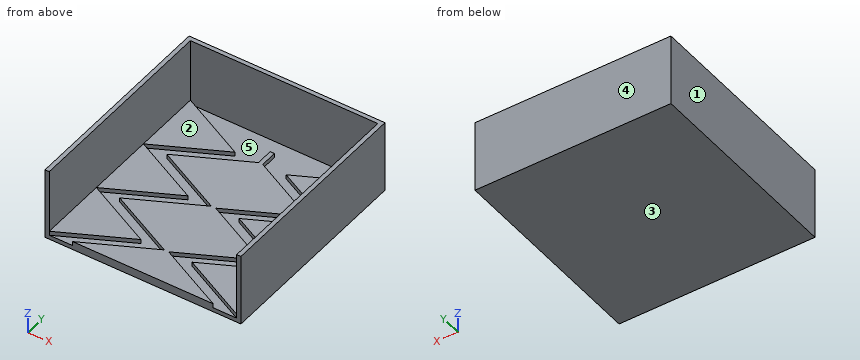
from build123d import *

# Parameters (mm, degrees)
F1_DEPTH = 3.175
F2_DEPTH = 50.8
F3_DEPTH = 3.175


# Not quite as in the source:
# - a length typed as a fraction of an inch, garbled in the dataset ("3 / 203.2 mm" for 3/8 in), is restored


with BuildPart() as f1:
    # F0 (on Top) → F1 (new body)
    with BuildSketch(Plane.XY):
        Polygon((53.975, 25.4), (3.175, 0), (20.638, 0), (71.438, 25.39975), (20.638, 50.7995), (71.438, 76.1995), (20.638, 101.5995), (71.438, 126.9995), (71.438, 139.6995), (74.613, 139.6995), (74.613, 126.9995), (125.412, 101.6), (74.612, 76.2), (125.412, 50.8), (74.612, 25.4), (125.412, 0), (142.875, 0), (92.075, 25.4), (142.875, 50.8), (92.075, 76.2), (142.875, 101.6), (92.075, 127), (142.875, 152.4), (3.175, 152.4), (53.975, 127), (3.175, 101.6), (53.975, 76.2), (3.175, 50.8), align=None)
        Polygon((142.875, 101.6), (142.875, 152.4), (92.075, 127), align=None)
        Polygon((0, 155.575), (0, 0), (3.175, 0), (3.175, 50.8), (3.175, 101.6), (3.175, 152.4), (142.875, 152.4), (142.875, 101.6), (142.875, 50.8), (142.875, 0), (146.05, 0), (146.05, 155.575), align=None)
        Polygon((92.075, 76.2), (142.875, 50.8), (142.875, 101.6), align=None)
        Polygon((92.075, 25.4), (142.875, 0), (142.875, 50.8), align=None)
        Polygon((71.438, 25.39975), (20.638, 0), (125.412, 0), (74.612, 25.4), (125.412, 50.8), (74.612, 76.2), (125.412, 101.6), (74.613, 126.9995), (74.613, 139.6995), (71.438, 139.6995), (71.438, 126.9995), (20.638, 101.5995), (71.438, 76.1995), (20.638, 50.7995), align=None)
        Polygon((3.175, 50.8), (3.175, 0), (53.975, 25.4), align=None)
        Polygon((3.175, 101.6), (3.175, 50.8), (53.975, 76.2), align=None)
        Polygon((3.175, 152.4), (3.175, 101.6), (53.975, 127), align=None)
    extrude(amount=-F1_DEPTH)

    # F0 (on Top) → F2 (join)
    with BuildSketch(Plane.XY):
        Polygon((0, 155.575), (0, 0), (3.175, 0), (3.175, 50.8), (3.175, 101.6), (3.175, 152.4), (142.875, 152.4), (142.875, 101.6), (142.875, 50.8), (142.875, 0), (146.05, 0), (146.05, 155.575), align=None)
    extrude(amount=F2_DEPTH)

    # F0 (on Top) → F3 (join)
    with BuildSketch(Plane.XY):
        Polygon((3.175, 152.4), (3.175, 101.6), (53.975, 127), align=None)
        Polygon((3.175, 101.6), (3.175, 50.8), (53.975, 76.2), align=None)
        Polygon((3.175, 50.8), (3.175, 0), (53.975, 25.4), align=None)
        Polygon((92.075, 25.4), (142.875, 0), (142.875, 50.8), align=None)
        Polygon((92.075, 76.2), (142.875, 50.8), (142.875, 101.6), align=None)
        Polygon((142.875, 101.6), (142.875, 152.4), (92.075, 127), align=None)
        Polygon((71.438, 25.39975), (20.638, 0), (125.412, 0), (74.612, 25.4), (125.412, 50.8), (74.612, 76.2), (125.412, 101.6), (74.613, 126.9995), (74.613, 139.6995), (71.438, 139.6995), (71.438, 126.9995), (20.638, 101.5995), (71.438, 76.1995), (20.638, 50.7995), align=None)
    extrude(amount=F3_DEPTH)


solid = f1.part
For this review, take the finished solid that the model builds, in its own axes (mm). Face numbers are marked on the shaded views. A direction names the side the tool comes from. Give positions to 0.01 mm unless a question says otherwise; leave off trailing zeros. Order: outer loops, then holes, each group sorted by start corner. A loop starts at its lowest first (then second) coordinate and runs counter-clockwise, first axis right, second up. Notation, with made-up numbers: M 17,20 L 67,20 A15 ccw 67,29 Z; hole C 3,21.25 d9. An arc over 180 degrees is marked long. Answer in a Markdown table with one row per item. Add a question column.
(1) Consider section C-C on x = 46. State the section outline as (y, z) points (1 decimal), and give its area (3 significant figures).
(2) For pin 1 (6 mm diameter, centred on y = 60.5, z = 18, fed in from -X); pin 2 (10 mm diameter, centred on x = 81, z = 19, fed in from -Y); pin 3 (15 mm diameter, centred on x = 113.5, y = 28.5, fed in from +Z) (3 decimals), all flat-tipped, find the tip position at first contact; note any pin that passes through.
(3) Consider section B-B on y = 111.5. State the section outline as (x, z) points (3 decimals).
(4) Mouldability with a two-part tool opening along Y and no side actions: class the marked faces 3, 4 and 5 as +Y half, -Y half, draft (parallel to the pull), parting line (faces both ways), or undercut.
(5) For the marked faces 1 and 2, list the 3-axis set-ups (+Z, -Z, +X, -X, +Y, -Y) from which the entire face can be reached by the end or side of a thin tool; tool diameter is ignored.
(6) Consider section A-A on z = 13. State the section outline as (x, y) points (3 decimals), and give its area (3 significant figures).
(7) Consider section D-D on y = 92. State the section outline as (x, z) points (3 decimals).
(8) Wall thickness on probe 1 along X at (y, z) = (47, 24.5) (3 decimals); probe 2 along Z at (x, y) = (117, 17.5) (3 decimals); probe 3 along Y at (x, z) = (80, 13.5) (3 decimals): over which ranges is each line inside the solid? List them lowest first. Write a range as [from, to].
Evaluation:
| question | item | result |
|---|---|---|
| 1 | outline | M 0,-3.2 L 155.6,-3.2 L 155.6,50.8 L 152.4,50.8 L 152.4,0 L 131,0 L 131,3.2 L 123,3.2 L 123,0 L 114.3,0 L 114.3,3.2 L 88.9,3.2 L 88.9,0 L 80.2,0 L 80.2,3.2 L 72.2,3.2 L 72.2,0 L 63.5,0 L 63.5,3.2 L 38.1,3.2 L 38.1,0 L 29.4,0 L 29.4,3.2 L 21.4,3.2 L 21.4,0 L 12.7,0 L 12.7,3.2 L 0,3.2 Z |
| 1 | area | 933 mm^2 |
| 2 | pin 1 | stops at x = 0 |
| 2 | pin 2 | stops at y = 152.4 |
| 2 | pin 3 | stops at z = 3.175 |
| 3 | outline | M 0,-3.175 L 146.05,-3.175 L 146.05,50.8 L 142.875,50.8 L 142.875,3.175 L 123.075,3.175 L 123.075,0 L 105.612,0 L 105.612,3.175 L 40.439,3.175 L 40.439,0 L 22.975,0 L 22.975,3.175 L 3.175,3.175 L 3.175,50.8 L 0,50.8 Z |
| 4 | face 3 | draft |
| 4 | face 4 | +Y half |
| 4 | face 5 | undercut |
| 5 | face 1 | +Z, -Z, -X, +Y, -Y |
| 5 | face 2 | +Z, -Y |
| 6 | outline | M 0,0 L 3.175,0 L 3.175,152.4 L 142.875,152.4 L 142.875,0 L 146.05,0 L 146.05,155.575 L 0,155.575 Z |
| 6 | area | 1,430 mm^2 |
| 7 | outline | M 0,-3.175 L 146.05,-3.175 L 146.05,50.8 L 142.875,50.8 L 142.875,3.175 L 123.675,3.175 L 123.675,0 L 106.212,0 L 106.212,3.175 L 39.837,3.175 L 39.837,0 L 22.375,0 L 22.375,3.175 L 3.175,3.175 L 3.175,50.8 L 0,50.8 Z |
| 8 | probe 1 | x = [0, 3.175], [142.875, 146.05] |
| 8 | probe 2 | z = [-3.175, 3.175] |
| 8 | probe 3 | y = [152.4, 155.575] |
